The listing builds one solid part. Answer for the finished solid, in the listing's coordinates (mm). Face numbers are marked on the shaded views. Coordinates: 2 decimals unless noted, no trailing zeros. Order: outer loops, then holes, each group sorted by start corner. A loop starts at its lowest first (then second) coordinate and runs counter-clockwise, first axis right, second up.
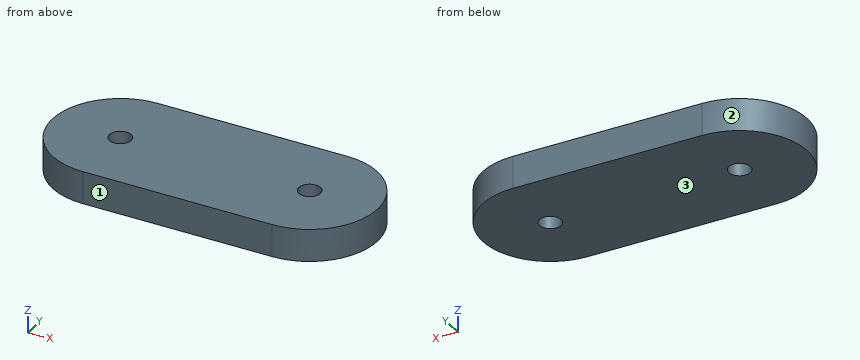
Autodesk Inventor part; units mm, degrees
ref_plane "YZ Plane" through (0, 0, 0) normal (1, 0, 0) x (0, 1, 0)
ref_plane "XZ Plane" through (0, 0, 0) normal (0, 1, 0) x (-1, 0, 0)
ref_plane "XY Plane" through (0, 0, 0) normal (0, 0, 1) x (1, 0, 0)
sketch "Sketch1" plane through (0, 0, 0) normal (0, 0, 1) x (1, 0, 0)
  line L0 (0, 0) -> (-60, 0)
  line L1 (-60, 0) -> (-60, 25)
  line L2 (-60, 25) -> (0, 25)
  line L3 (0, 25) -> (0, 0)
  dimension "d0" = 60
  dimension "d1" = 25
extrude "Extrusion3" add sketch "Sketch1" along normal blind 6
sketch "Sketch3" plane through (0, 0, 6) normal (0, 0, 1) x (1, 0, 0)
  circle A0 centre (-47.5, 12.5) radius 12.5
  line L0 (-60, 0) -> (0, 0)
  line L1 (-60, 25) -> (-60, 0)
  circle A1 centre (-12.5, 12.5) radius 12.5
  line L2 (0, 25) -> (-60, 25)
  line L3 (0, 0) -> (0, 25)
  circle A2 centre (-47.5, 12.5) radius 2
  circle A3 centre (-12.5, 12.5) radius 2
  point P0 (0, 12.5)
  point P1 (-12.5, 0)
  point P2 (-12.5, 25)
  point P3 (-47.5, 25)
  point P4 (-60, 12.5)
  point P5 (-47.5, 0)
  dimension "d16" = 25
  dimension "d17" = 12.5
  dimension "d18" = 12.5
  dimension "d19" = 25
  dimension "d20" = 12.5
  dimension "d21" = 12.5
  dimension "d22" = 4
  dimension "d23" = 4
extrude "Extrusion4" cut sketch "Sketch3" against normal blind 6 contours A0 L1 L2 | L0 L1 A0 | L2 L3 A1 | A1 L3 L0 | A2 | A3
properties part number "Middle"
(1) Find section B-B (z = 1.6). Write down the section's boundary in (x, y).
(2) Find section D-D (x = -8). Write down the section's boundary in (y, z), and give its area (3 significant figures).
(3) The mould has two halves that part along Y. Classify the marked faces 1, 2 and 3: released by +Y, released by -Y, zero draft, split by the parting line, or undercut.
(4) Find section C-C (y = 2.5). Write down the section's boundary in (x, z).
(5) Find section A-A (y = 12.5). Write down the section's boundary in (x, z), and give its area (3 significant figures).
(6) Consider line 1 (Y direction, x = -47.5, z = 2.85); line 2 (X direction, y = 10.75, z = 3.85); line 3 (Y direction, x = -8, z = 2.45). Determine where each line is inside the solid, lowest interval first.
Findings below:
1. outline: (-47.5, 0) - (-12.5, 0) arc R12.5 ccw to (-12.5, 25) - (-47.5, 25) arc R12.5 ccw to start; hole circle Ø4 at (-47.5, 12.5); hole circle Ø4 at (-12.5, 12.5)
2. outline: (0.84, 0) - (24.16, 0) - (24.16, 6) - (0.84, 6) - close
2. area: 140 mm2
3. face 1: released by -Y
3. face 2: split by the parting line
3. face 3: zero draft
4. outline: (-55, 0) - (-5, 0) - (-5, 6) - (-55, 6) - close
5. outline: (-60, 0) - (-49.5, 0) - (-49.5, 6) - (-60, 6) - close; (-45.5, 0) - (-14.5, 0) - (-14.5, 6) - (-45.5, 6) - close; (-10.5, 0) - (0, 0) - (0, 6) - (-10.5, 6) - close
5. area: 312 mm2
6. line 1: y = 0 to 10.5, 14.5 to 25
6. line 2: x = -59.88 to -48.47, -46.53 to -13.47, -11.53 to -0.12
6. line 3: y = 0.84 to 24.16
